```python
from build123d import *

# Parameters (mm, degrees)
SKETCH1_R           = 1524
SKETCH1_R_2         = 762
EXTRUDE_THIN1_DEPTH = 1778
SKETCH2_W           = 25.4
SKETCH2_H           = 127
CUT_EXTRUDE1_DEPTH  = 2795
CIRPATTERN1_COUNT   = 20
SCALE1_SCALE        = 0.02


with BuildPart() as part:
    # Sketch1 → Extrude-Thin1 (new body)
    with BuildSketch(Plane(origin=(0, 0, 0), x_dir=(1, 0, 0), z_dir=(0, 1, 0))):
        Circle(SKETCH1_R)
        Circle(SKETCH1_R_2, mode=Mode.SUBTRACT)
    extrude(amount=EXTRUDE_THIN1_DEPTH)

    # Sketch2 → Cut-Extrude1 (cut, through all)
    with BuildSketch(Plane(origin=(0, 1778, 0), x_dir=(1, 0, 0), z_dir=(0, 1, 0))):
        with Locations((0, 762)):
            Rectangle(SKETCH2_W, SKETCH2_H)
    cut_extrude1 = extrude(amount=-CUT_EXTRUDE1_DEPTH, mode=Mode.SUBTRACT)

    # CirPattern1: Cut-Extrude1 ×20 about axis
    cirpattern1_axis = Axis((0, 0, 0), (0, 1, 0))
    for i in range(1, CIRPATTERN1_COUNT):
        add(cut_extrude1.rotate(cirpattern1_axis, i * 360 / CIRPATTERN1_COUNT), mode=Mode.SUBTRACT)


with BuildPart() as part_1:
    # Scale1: scaled about (0, 889, 0)
    add(part.part.scale(SCALE1_SCALE).moved(Location((0, 871.22, 0))))


solid = part_1.part
```
Can you work these out from the model? Positions are in its coordinate system, mm. Give positions to 0.01 mm unless a question says otherwise; leave off trailing zeros. Write item = value, one per line. Start each with the question number.
Q1. Will these pins go through, and if not, where does the flat tip stop? pin 1 Ø1.4 at (y, z) = (888.5, -15.5) entering from +X; pin 2 Ø1 at (x, y) = (-16, 881.5) entering from +Z; pin 3 Ø8 at (x, y) = (17, 883.5) entering from -Z.
Q2. We'd pull the mould along X, two halves only. Please class faces 1 (the cylindrical face through (-6.607, 888.751, 29.755)), 2 (the cylindrical face through (-6.945, 888.751, 13.565)), 3 (the cylindrical face through (-15.05, 888.75, -2.41)), 4 (the flat face through (-7, 871.22, -14)): pulls with the +X half, pulls with the -X half, needs draft (parallel to the pull), parting line crosses it, or undercut.
Q3. I need wall thicknesses on probe 1 along X at (y, z) = (898, 0); probe 2 along X at (y, z) = (904, -13); probe 3 along Z at (x, y) = (-9, 903.5). Which ranges of each line are inside material? Lowest first, please. Write a range as [from, to].
Check result:
q1.pin_1 = 26.65
q1.pin_2 = 26.24
q1.pin_3 = -27.57
q2.face_1 = parting line crosses it
q2.face_2 = undercut
q2.face_3 = undercut
q2.face_4 = needs draft
q3.probe_1 = [-30.48, -16.51], [16.51, 30.48]
q3.probe_2 = [-27.57, -9.76], [-9.13, -7.95], [7.95, 9.13], [9.76, 27.57]
q3.probe_3 = [-29.12, -12.82], [12.82, 29.12]
